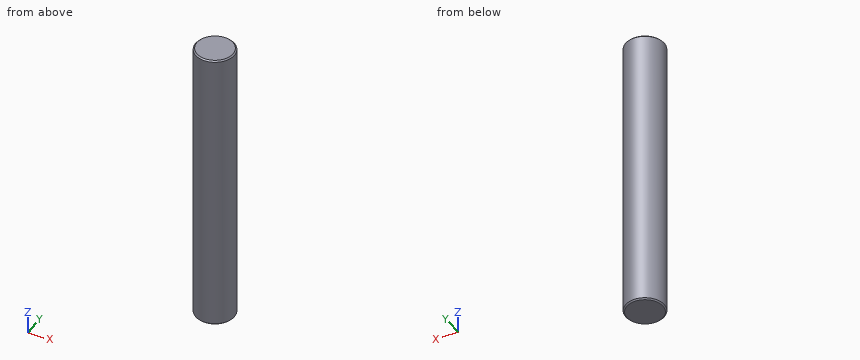
```python
from build123d import *

# Parameters (mm, degrees)
SKETCH_R        = 3
PAD_DEPTH       = 45
CHAMFER_SIZE    = 0.2
CHAMFER001_SIZE = 0.2


with BuildPart() as part:
    # Sketch → Pad (new body)
    with BuildSketch(Plane.XY):
        Circle(SKETCH_R)
    extrude(amount=PAD_DEPTH)

    # Chamfer
    chamfer_edges = [part.edges().sort_by_distance(p)[0] for p in [
        (-3, 0, 45),
    ]]
    chamfer(chamfer_edges, length=CHAMFER_SIZE)

    # Chamfer001
    chamfer001_edges = [part.edges().sort_by_distance(p)[0] for p in [
        (-3, 0, 0),
    ]]
    chamfer(chamfer001_edges, length=CHAMFER001_SIZE)


solid = part.part
```
Could you check a few things on this model? Use its own coordinates, in mm. Give positions to 0.01 mm unless a question says otherwise; leave off trailing zeros. Loops run counter-clockwise (first coordinate to the right, second up) from the corner with the lowest first, then second, coordinate; pieces in that order, holes last. Notation, with made-up numbers: (49, -26) - (55, -26) arc R22 ccw to (55, -15) - close; hole circle Ø9 at (27.25, 72.25). An arc over 180 degrees is marked (long way). Answer in a Markdown table with one row per item. Add a question column.
Q1. If we section it at A-A (z = 32.5): List the corners of the cut face in (x, y) for me, plus the area to 3 significant figures.
Q2. Please list where these lines run through material, in increasing order: L1, parallel to X at y = 0.2, z = 9; L2, parallel to X at y = -1.2, z = 32; L3, parallel to Y at x = -2.55, z = 7. Write a range as from..to.
Q3. For pin 1 (1.5 mm diameter, centred on x = 2, z = 11.5, fed in from -Y), with a flat end and sliding along its axis, tell me the tip position at first contact or that it passes through.
The answers:
| question | item | result |
|---|---|---|
| 1 | outline | circle Ø6 at (0, 0) |
| 1 | area | 28.3 mm^2 |
| 2 | L1 | x = -2.99..2.99 |
| 2 | L2 | x = -2.75..2.75 |
| 2 | L3 | y = -1.58..1.58 |
| 3 | pin 1 | stops at y = -2.73 |
